Answer from the drawing. Dimensions are ordinates in mm from the lowest x, y and z of the part. A direction names the side the tool comes from. Coordinates: 2 decimals unless noted, no trailing zeros. Loops run counter-clockwise (first coordinate to the right, second up) from the corner with the lowest first, then second, coordinate; pieces in that order, holes last. Notation, with made-up numbers: (-24.75, -6) - (17.25, -6) arc R16 ccw to (17.25, 18) - close; hole circle Ø2 at (-6, 6). An arc over 180 degrees is marked (long way). Write each question's results on one line, items separated by ' | '. Start each with the question number.
1. A cutting plane is placed at D-D on z = 10. Determine the outline of the cut face in (x, y).
2. A cutting plane is placed at A-A on z = 2. Determine the outline of the cut face in (x, y).
3. Which of the six approach directions +Z, -Z, +X, -X, +Y, -Y give full straight-line access (tool end or side, diameter ignored) to the marked faces 4, 5 and 6?
4. A cutting plane is placed at C-C on y = 1.9. State how many separate pieces and enclosed holes the cut face has, then the cut area to 3 significant figures.
5. A cutting plane is placed at B-B on x = 18. Determine the outline of the cut face in (y, z), then the cut area to 3 significant figures.
6. Each of these flat-tipped pins is pushed along its axis until it touches: P1, Ø2.5, axis at x = 15.66, z = 4.34, coming from the +Y side; P2, Ø2, axis at x = 16.5, y = 2, coming from the -Z side; P3, Ø1.8, axis at x = 10, z = 2, coming from the +Y side; P4, Ø2, axis at y = 3, z = 8, coming from the -X side. Where does it stop, or does it pass through?
7. Determine the mould class of the marked faces 1, 2 and 3 for opening direction Z: released by +Z, released by -Z, zero draft, split by the parting line, or undercut.
8. Find the intervals of material crossed by line 1 along Z through (x, y) = (10, 1.65); line 2 along Z through (x, y) = (5, 2.95); line 3 along Y through (x, z) = (14.5, 13.75), in increasing order. Write a range as [from, to].
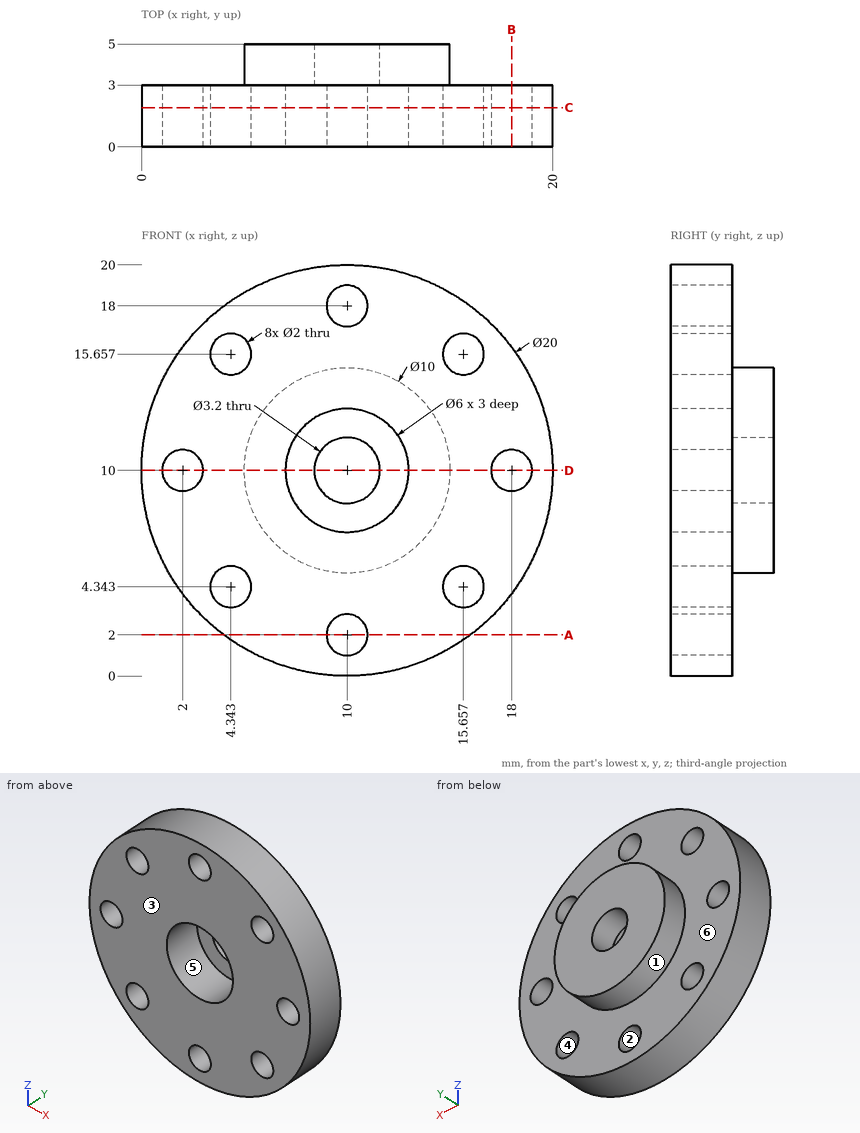
Values:
1) outline: (0, 0) - (1, 0) - (1, 3) - (0, 3) - close; (3, 0) - (7, 0) - (7, 3) - (8.4, 3) - (8.4, 5) - (5, 5) - (5, 3) - (3, 3) - close; (11.6, 3) - (13, 3) - (13, 0) - (17, 0) - (17, 3) - (15, 3) - (15, 5) - (11.6, 5) - close; (19, 0) - (20, 0) - (20, 3) - (19, 3) - close
2) outline: (4, 0) - (9, 0) - (9, 3) - (4, 3) - close; (11, 0) - (16, 0) - (16, 3) - (11, 3) - close
3) face 4: +Y, -Y | face 5: -Y | face 6: +Y
4) separate pieces: 1 | enclosed holes: 9 | area: 261 mm^2
5) outline: (0, 4) - (3, 4) - (3, 9) - (0, 9) - close; (0, 11) - (3, 11) - (3, 16) - (0, 16) - close | area: 30.0 mm^2
6) P1: y = 3 | P2: z = 1.65 | P3: through | P4: x = 0.05
7) face 1: split by the parting line | face 2: undercut | face 3: zero draft
8) line 1: [0, 1], [3, 7], [13, 17], [19, 20] | line 2: [1.34, 3.59], [5.1, 14.9], [16.41, 18.66] | line 3: [0, 3]
